Design review of the part built by this model. Coordinates are the model's own, in mm. Round coordinates to 2 decimals unless told otherwise and drop trailing zeros. Write each loop counter-clockwise with the first axis right and the second up, starting at its lowest first coordinate (ties: lowest second). Pieces come first, ordered by that corner, then holes. Notation, with made-up numbers: M 15,40.5 L 21,40.5 A27 cw 21,74.5 Z; hole C 24.5,-7.5 d8. An arc over 180 degrees is marked long. Use CSV: the item, a comma, the result in double quotes.
from build123d import *

# Parameters (mm, degrees)
SKETCH1_W           = 114.7953
SKETCH1_H           = 19.1516
SKETCH1_W_2         = 19.1516
BOSS_EXTRUDE1_DEPTH = 1.8288


with BuildPart() as part:
    # Sketch1 → Boss-Extrude1 (new body)
    with BuildSketch(Plane(origin=(0, 0, 0), x_dir=(0, 0, -1), z_dir=(1, 0, 0))):
        Polygon((-31.179336382, -25.30028674), (-31.179336382, 22.47711326), (-31.179336382, 41.62871326), (-50.330936382, 41.62871326), (-50.330936382, -25.30028674), align=None)
        with Locations((26.218313618, 32.05291326)):
            Rectangle(SKETCH1_W, SKETCH1_H)
        with Locations((26.218313618, -34.87608674)):
            Rectangle(SKETCH1_W, SKETCH1_H)
        with Locations((-40.755136382, -34.87608674)):
            Rectangle(SKETCH1_W_2, SKETCH1_H)
    extrude(amount=BOSS_EXTRUDE1_DEPTH)


solid = part.part
1) Add section C-C on y = -17. Write out the cut boundary in (x, z), then the cut area to 3 significant figures.
Answers:
outline,"M 0,31.18 L 1.83,31.18 L 1.83,50.33 L 0,50.33 Z"
area,"35.0 mm²"
2) For pin 1 Ø0.5 at (x, y) = (1, -3.5) entering from -Z; pin 2 Ø10 at (y, z) = (-31, -59) entering from -X, all flat-tipped, find the tip position at first contact; note any pin that passes through.
Answers:
pin 1,"z = 31.18"
pin 2,"x = 0"
3) Wall thickness on line 1 along Y through (x, z) = (1.4, 10.5); line 2 along Z through (x, y) = (1.4, -7.5): over which ranges is each line inside the solid? List them lowest first. Write a range as [from, to].
Answers:
line 1,"[-44.45, -25.3], [22.48, 41.63]"
line 2,"[31.18, 50.33]"
4) Add section B-B on x = 0.4. Write out the cut boundary in (y, z), then the cut area to 3 significant figures.
Answers:
outline,"M -44.45,-83.62 L -25.3,-83.62 L -25.3,31.18 L 22.48,31.18 L 22.48,-83.62 L 41.63,-83.62 L 41.63,50.33 L -44.45,50.33 Z"
area,"6,050 mm²"
5) Add section A-A on z = 23.5. Write out the cut boundary in (x, y).
Answers:
outline,"M 0,-44.45 L 1.83,-44.45 L 1.83,-25.3 L 0,-25.3 Z; M 0,22.48 L 1.83,22.48 L 1.83,41.63 L 0,41.63 Z"
